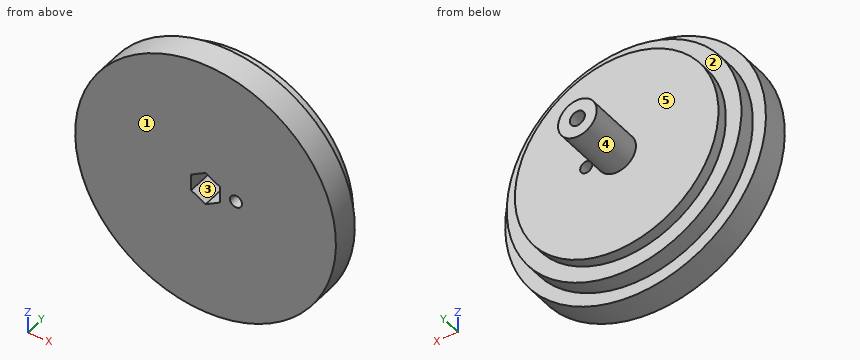
from build123d import *

# Parameters (mm, degrees)
CUT_EXTRUDE2_REACH    = 46.286
SKETCH3_R             = 1.397
SKETCH12_R            = 4.445
BOSS_EXTRUDE1_DEPTH   = 13.208
F_4_CLEARANCE_HOLE1_D = 3.4544
CUT_EXTRUDE3_DEPTH    = 8.5


with BuildPart() as part:
    # Sketch1 → Revolve1 (revolve)
    with BuildSketch(Plane.XY, mode=Mode.PRIVATE) as revolve1_sk:
        Polygon((0, 0), (-23.425, 0), (-23.425, -2.5), (-27, -2.5), (-27, -6.35), (-30, -6.35), (-30, -12.7), (0, -12.7), align=None)
    revolve(revolve1_sk.sketch.rotate(Axis((0, -12.7, 0), (0, 1, 0)), 270), axis=Axis((0, -12.7, 0), (0, 1, 0)))

    # Sketch3 → Cut-Extrude2 (cut, up to next)
    with BuildSketch(Plane.XZ, mode=Mode.PRIVATE) as cut_extrude2_sk1:
        with Locations(Location((7, 0, 0), (0, 0, 90))):
            Circle(SKETCH3_R)
    cut_extrude2_tool1 = extrude(cut_extrude2_sk1.sketch, amount=CUT_EXTRUDE2_REACH, mode=Mode.PRIVATE) & part.part
    add(cut_extrude2_tool1.solids().sort_by_distance((7, 0, 0))[0], mode=Mode.SUBTRACT)

    # Sketch12 → Boss-Extrude1 (add)
    with BuildSketch(Plane(origin=(0, 0, 0), x_dir=(1, 0, 0), z_dir=(0, 1, 0))):
        with Locations(Location((0, 0, 0), (0, 0, 90))):
            Circle(SKETCH12_R)
    extrude(amount=BOSS_EXTRUDE1_DEPTH)

    # #4 Clearance Hole1 (through all)
    with Locations(Plane(origin=(0, 13.208, 0), x_dir=(1, 0, 0), z_dir=(0, 1, 0))):
        with Locations((0, 0)):
            Hole(F_4_CLEARANCE_HOLE1_D / 2)

    # Sketch15 → Cut-Extrude3 (cut)
    with BuildSketch(Plane(origin=(0, -12.7, 0), x_dir=(-1, 0, 0), z_dir=(0, -1, 0))):
        Polygon((0, -3.812821178), (3.302, -1.906410589), (3.302, 1.906410589), (0, 3.812821178), (-3.302, 1.906410589), (-3.302, -1.906410589), align=None)
    extrude(amount=-CUT_EXTRUDE3_DEPTH, mode=Mode.SUBTRACT)


solid = part.part
CAD build for the part. Positions are in the model's coordinates, mm. Face numbers are marked on the shaded views. A direction names the side the tool comes from. Round coordinates to 2 decimals unless told otherwise and drop trailing zeros. Write each loop counter-clockwise with the first axis right and the second up, starting at its lowest first coordinate (ties: lowest second). Pieces come first, ordered by that corner, then holes. Notation, with made-up numbers: M -1.75,-33 L 42.25,-33 A30 cw 42.25,3 Z; hole C 58.5,70 d5. An arc over 180 degrees is marked long. Use a Markdown table: item, result. Add a question column.
1. Drill centre lines: probe 1 along X at (y, z) = (-10, 0); probe 2 along Y at (x, z) = (-8, 6); probe 3 along Y at (x, z) = (-17, -22.5). Where is each one in solid material? Low to high.
2. Flat gauge pins, fed straight in: P1, Ø5, axis at y = -8, z = 13, coming from the +X side; P2, Ø4, axis at y = -10, z = 0, coming from the +X side; P3, Ø10, axis at y = 6, z = 6.5, coming from the -X side; P4, Ø10, axis at x = -5.5, z = -2.5, coming from the +Y side. Where does each tip first touch, or does it go through?
3. Slice it at B-B on y = -9.25. Give the cut face in (x, z), then the cut area to 3 significant figures.
4. Slice it at D-D on z = 14.5. Give the cut face in (x, y), then the cut area to 3 significant figures.
5. 3-axis set-ups, long thin cutter, end or side, ignore diameter. For the marked faces 1 and 2: which of +Z, -Z, +X, -X, +Y, -Y reach the whole face in a straight line?
6. Slice it at C-C on y = 2. Give the cut face in (x, z) (3 decimals), then the cut area to 3 significant figures.
7. Pull direction Z, two halves, no side cores. Call the marked faces 3, 4 and 5: released by +Z, released by -Z, zero draft, split by the parting line, or undercut.
8. Slice it at A-A on z = 0. Give the cut face in (x, y) (3 decimals), then the cut area to 3 significant figures.
Reply:
| question | item | result |
|---|---|---|
| 1 | probe 1 | x = -30 to -3.3, 3.3 to 5.6, 8.4 to 30 |
| 1 | probe 2 | y = -12.7 to 0 |
| 1 | probe 3 | y = -12.7 to -6.35 |
| 2 | P1 | stops at x = 28.1 |
| 2 | P2 | stops at x = 30 |
| 2 | P3 | stops at x = -4.18 |
| 2 | P4 | stops at y = 13.21 |
| 3 | outline | C 0,0 d60; hole M -3.3,-1.91 L 0,-3.81 L 3.3,-1.91 L 3.3,1.91 L 0,3.81 L -3.3,1.91 Z; hole C 7,0 d2.79 |
| 3 | area | 2,780 mm^2 |
| 4 | outline | M -26.26,-12.7 L 26.26,-12.7 L 26.26,-6.35 L 22.78,-6.35 L 22.78,-2.5 L 18.4,-2.5 L 18.4,0 L -18.4,0 L -18.4,-2.5 L -22.78,-2.5 L -22.78,-6.35 L -26.26,-6.35 Z |
| 4 | area | 601 mm^2 |
| 5 | face 1 | +Z, -Z, +X, -X, -Y |
| 5 | face 2 | +Y |
| 6 | outline | C 0,0 d8.89; hole C 0,0 d3.454 |
| 6 | area | 52.7 mm^2 |
| 7 | face 3 | undercut |
| 7 | face 4 | split by the parting line |
| 7 | face 5 | zero draft |
| 8 | outline | M -30,-12.7 L -3.302,-12.7 L -3.302,-4.2 L -1.727,-4.2 L -1.727,13.208 L -4.445,13.208 L -4.445,0 L -23.425,0 L -23.425,-2.5 L -27,-2.5 L -27,-6.35 L -30,-6.35 Z; M 1.727,-4.2 L 3.302,-4.2 L 3.302,-12.7 L 5.603,-12.7 L 5.603,0 L 4.445,0 L 4.445,13.208 L 1.727,13.208 Z; M 8.397,-12.7 L 30,-12.7 L 30,-6.35 L 27,-6.35 L 27,-2.5 L 23.425,-2.5 L 23.425,0 L 8.397,0 Z |
| 8 | area | 672 mm^2 |
